from build123d import *

# Parameters (mm, degrees)
SKETCH1_W           = 70
SKETCH1_H           = 54
BOSS_EXTRUDE1_DEPTH = 2
SKETCH2_W           = 5
SKETCH2_H           = 40
BOSS_EXTRUDE2_DEPTH = 1
BOSS_EXTRUDE3_START = -24
BOSS_EXTRUDE3_DEPTH = 6


with BuildPart() as part:
    # Sketch1 → Boss-Extrude1 (new body)
    with BuildSketch(Plane(origin=(0, 0, 0), x_dir=(1, 0, 0), z_dir=(0, 1, 0))):
        Rectangle(SKETCH1_W, SKETCH1_H)
    extrude(amount=BOSS_EXTRUDE1_DEPTH)

    # Sketch2 → Boss-Extrude2 (add)
    with BuildSketch(Plane.XZ):
        with Locations((-35, 0)):
            Rectangle(SKETCH2_W, SKETCH2_H)
    extrude(amount=BOSS_EXTRUDE2_DEPTH)

    # Sketch3 → Boss-Extrude3 (add)
    with BuildSketch(Plane.XY.offset(27).offset(BOSS_EXTRUDE3_START)):
        Polygon((35.85458287, -3.981493023), (39.307999477, 2), (32.401166263, 2), align=None)
    extrude(amount=-BOSS_EXTRUDE3_DEPTH)


solid = part.part
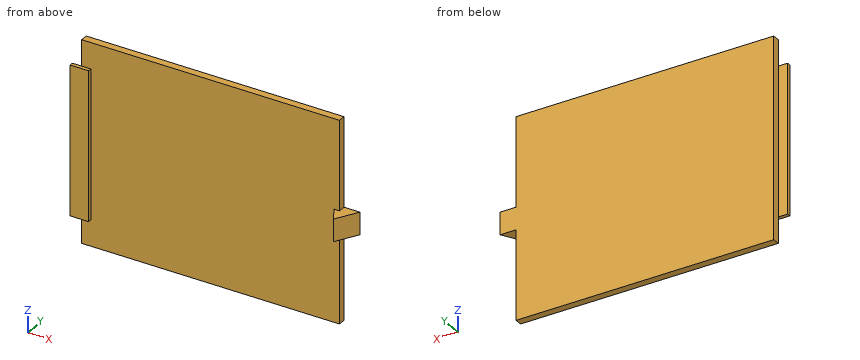
Design review of the part built by this model. Coordinates are the model's own, in mm. Give positions to 0.01 mm unless a question says otherwise; leave off trailing zeros. Order: outer loops, then holes, each group sorted by start corner. A loop starts at its lowest first (then second) coordinate and runs counter-clockwise, first axis right, second up. Notation, with made-up numbers: (-11, 76.5) - (7, 76.5) arc R29 ccw to (7, 112.5) - close; hole circle Ø8 at (-17, 54). An arc over 180 degrees is marked (long way). Use CSV: the item, a comma, the result in double quotes. Start each with the question number.
Q1. For line 1 (Y direction, x = -19, z = 5.5); line 2 (X direction, y = 1.25, z = -22), list the stretches that pass through material, from the lowest coordinate up.
Q2. Take a section at A-A (z = -14). State the section outline as (x, y) points.
Q3. Take a section at D-D (z = -0.5). State the section outline as (x, y) points, and give its area (3 significant figures).
Q4. Take a section at B-B (x = -6). State the section outline as (y, z) points, and give its area (3 significant figures).
Q5. Take a section at C-C (y = 1.1). State the section outline as (x, z) points.
Q6. For P1, Ø3, axis at x = -25.5, y = -1, coming from the +Z side; P2, Ø0.5, axis at x = -35.5, y = -0.5, coming from the +Z side; P3, Ø1.1, axis at y = -0.5, z = 9, coming from the +X side; P4, Ø1.5, axis at x = 17.5, z = -10, coming from the -Y side, all flat-tipped, find the tip position at first contact; note any pin that passes through.
Calculated:
1,line 1,"y = 0 to 2"
1,line 2,"x = -35 to 35"
2,outline,"(-37.5, -1) - (-32.5, -1) - (-32.5, 0) - (35, 0) - (35, 2) - (-35, 2) - (-35, 0) - (-37.5, 0) - close"
3,outline,"(-37.5, -1) - (-32.5, -1) - (-32.5, 0) - (33.56, 0) - (35.85, -3.98) - (39.31, 2) - (-35, 2) - (-35, 0) - (-37.5, 0) - close"
3,area,"162 mm²"
4,outline,"(0, -27) - (2, -27) - (2, 27) - (0, 27) - close"
4,area,"108 mm²"
5,outline,"(-35, -27) - (35, -27) - (35, -3) - (38.79, -3) - (38.79, 3) - (35, 3) - (35, 27) - (-35, 27) - close"
6,P1,"stops at z = 27"
6,P2,"stops at z = 20"
6,P3,"stops at x = 35"
6,P4,"stops at y = 0"
